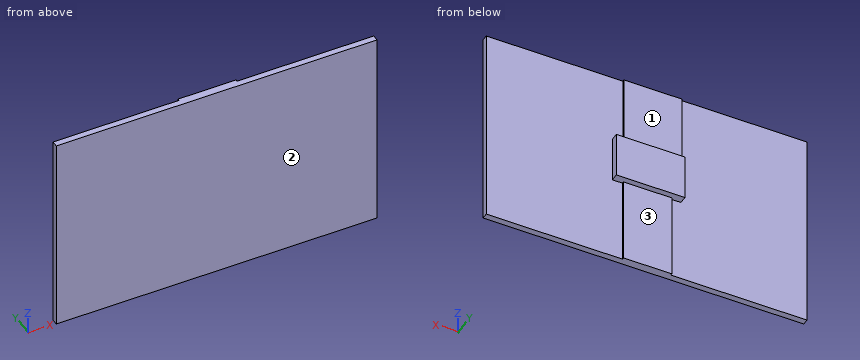
from build123d import *

# Parameters (mm, degrees)
SKETCH1_W           = 35.5
SKETCH1_H           = 24
BOSS_EXTRUDE1_DEPTH = 4
SKETCH1_3_W         = 25
SKETCH1_3_H         = 45
SKETCH1_3_W_2       = 30
SKETCH1_3_H_2       = 36.5
SKETCH1_3_W_3       = 35.5
SKETCH1_3_H_3       = 24
BOSS_EXTRUDE2_DEPTH = 3.2
SKETCH1_4_W         = 25
SKETCH1_4_H         = 45
SKETCH1_4_W_2       = 30
SKETCH1_4_H_2       = 36.5
BOSS_EXTRUDE3_DEPTH = 1


with BuildPart() as part:
    # Sketch1 → Boss-Extrude1 (new body)
    with BuildSketch(Plane(origin=(0, 0, 0), x_dir=(1, 0, 0), z_dir=(0, 1, 0))):
        with Locations((0, -4.25)):
            Rectangle(SKETCH1_W, SKETCH1_H)
    extrude(amount=BOSS_EXTRUDE1_DEPTH)

    # Sketch1_3 → Boss-Extrude2 (add)
    with BuildSketch(Plane(origin=(0, 0, 0), x_dir=(1, 0, 0), z_dir=(0, 1, 0))):
        Polygon((-12.5, 52.75), (-83, 52.75), (-83, -52.75), (-17.75, -52.75), (-17.75, -16.25), (-17.75, 7.75), (-12.5, 7.75), align=None)
        with Locations((0, 30.25)):
            Rectangle(SKETCH1_3_W, SKETCH1_3_H)
        with Locations((-2.75, -34.5)):
            Rectangle(SKETCH1_3_W_2, SKETCH1_3_H_2)
        Polygon((83, 52.75), (12.5, 52.75), (12.5, 7.75), (17.75, 7.75), (17.75, -16.25), (12.25, -16.25), (12.25, -52.75), (83, -52.75), align=None)
        with Locations((0, -4.25)):
            Rectangle(SKETCH1_3_W_3, SKETCH1_3_H_3)
    extrude(amount=-BOSS_EXTRUDE2_DEPTH)

    # Sketch1_4 → Boss-Extrude3 (add)
    with BuildSketch(Plane(origin=(0, 0, 0), x_dir=(1, 0, 0), z_dir=(0, 1, 0))):
        with Locations((0, 30.25)):
            Rectangle(SKETCH1_4_W, SKETCH1_4_H)
        with Locations((-2.75, -34.5)):
            Rectangle(SKETCH1_4_W_2, SKETCH1_4_H_2)
    extrude(amount=BOSS_EXTRUDE3_DEPTH)


solid = part.part
CAD build for the part. Positions are in the model's coordinates, mm. Face numbers are marked on the shaded views. A direction names the side the tool comes from. Coordinates: 2 decimals unless noted, no trailing zeros. Order: outer loops, then holes, each group sorted by start corner. A loop starts at its lowest first (then second) coordinate and runs counter-clockwise, first axis right, second up.
Item 1: Band-saw the part on D-D on x = 31. List the corners of the cut face in (y, z), plus the area to 3 significant figures.
Check sheet entries:
outline: (-3.2, -52.75) - (0, -52.75) - (0, 52.75) - (-3.2, 52.75) - close
area: 338 mm2
Item 2: Band-saw the part on A-A on z = 39. List the corners of the cut face in (x, y).
Check sheet entries:
outline: (-83, -3.2) - (83, -3.2) - (83, 0) - (12.25, 0) - (12.25, 1) - (-17.75, 1) - (-17.75, 0) - (-83, 0) - close
Item 3: 3-axis set-ups, long thin cutter, end or side, ignore diameter. For the marked faces 1, 2 and 3: which of +Z, -Z, +X, -X, +Y, -Y reach the whole face in a straight line?
Check sheet entries:
face 1: +Z, +X, -X, +Y
face 2: +Z, -Z, +X, -X, -Y
face 3: -Z, +X, -X, +Y
Item 4: Drill centre lines: L1, parallel to X at y = 1, z = -2; L2, parallel to Y at x = 25, z = -9; L3, parallel to Z at x = -13.5, y = 2. Where is each one in solid material? Low to high.
Check sheet entries:
L1: x = -17.75 to 17.75
L2: y = -3.2 to 0
L3: z = -7.75 to 16.25
Item 5: Band-saw the part on B-B on x = 8.5. List the corners of the cut face in (y, z), plus the area to 3 significant figures.
Check sheet entries:
outline: (-3.2, -52.75) - (1, -52.75) - (1, -7.75) - (4, -7.75) - (4, 16.25) - (1, 16.25) - (1, 52.75) - (-3.2, 52.75) - close
area: 515 mm2
Item 6: Pin check, flat tips, straight feed: pin 1 Ø1.5 at (y, z) = (1, 11) entering from -X; pin 2 Ø3 at (y, z) = (2.5, -1) entering from +X; pin 3 Ø0.8 at (y, z) = (0.5, -39.5) entering from +X. Stop position of each tip, or through.
Check sheet entries:
pin 1: stops at x = -17.75
pin 2: stops at x = 17.75
pin 3: stops at x = 12.5
Item 7: Band-saw the part on C-C on y = 2.25. List the corners of the cut face in (x, z), plus the area to 3 significant figures.
Check sheet entries:
outline: (-17.75, -7.75) - (17.75, -7.75) - (17.75, 16.25) - (-17.75, 16.25) - close
area: 852 mm2
